Design review of the part built by this model. Coordinates are the model's own, in mm. A direction names the side the tool comes from. Coordinates: 2 decimals unless noted, no trailing zeros. Loops run counter-clockwise (first coordinate to the right, second up) from the corner with the lowest first, then second, coordinate; pieces in that order, holes last. Notation, with made-up numbers: (15, 63.5) -> (19, 63.5) arc R25 ccw to (19, 97.5) -> close; hole circle Ø5 at (38.5, 15.25). An arc over 180 degrees is marked (long way). Answer as a JSON object with one key per item and string values.
Autodesk Inventor part; units mm, degrees
ref_plane "XZ Plane" through (0, 0, 0) normal (0, 1, 0) x (-1, 0, 0)
sketch "Sketch1" plane through (0, 0, 0) normal (0, 1, 0) x (-1, 0, 0)
  line L0 (0, -8.89) -> (0, 8.89)
  line L1 (-35.56, 0) -> (35.56, 0)
  line L2 (25.4, -6.35) -> (-25.4, -6.35)
  line L3 (-25.4, -6.35) -> (-25.4, 6.35)
  line L4 (-25.4, 6.35) -> (25.4, 6.35)
  line L5 (25.4, 6.35) -> (25.4, -6.35)
  point P0 (0, 0)
  dimension "d0" = 12.7
  dimension "d1" = 6.35
  dimension "d2" = 50.8
  dimension "d3" = 25.4
extrude "Extrusion1" add sketch "Sketch1" along normal blind 4.7625
sketch "Sketch2" plane through (0, 4.7625, 0) normal (0, 1, 0) x (1, 0, 0)
  line L0 (25.4, 6.35) -> (-25.4, 6.35)
  line L1 (-25.4, 6.35) -> (-25.4, -6.35)
  line L2 (-25.4, -6.35) -> (25.4, -6.35)
  line L3 (25.4, -6.35) -> (25.4, 6.35)
  line L4 (-25.4, 2.5146) -> (-12.855, 6.35)
  line L5 (25.4, 6.35) -> (-25.4, 6.35)
  line L6 (-25.4, 6.35) -> (-25.4, -6.35)
  line L7 (-25.4, -2.5146) -> (-12.855, -6.35)
  line L8 (-12.855, 6.35) -> (-12.855, -6.35) construction
  line L9 (0, 8.89) -> (0, -8.89)
  line L10 (35.56, 0) -> (-35.56, 0)
  line L11 (-1.5875, 2.2479) -> (19.05, 2.2479)
  line L12 (19.05, 2.2479) -> (19.05, -2.2479)
  line L13 (19.05, -2.2479) -> (-1.5875, -2.2479)
  line L14 (-1.5875, -2.2479) -> (-1.5875, 2.2479)
  circle A0 centre (19.05, 0) radius 2.2479
  circle A1 centre (-1.5875, 0) radius 2.2479
  point P0 (0, 0)
  dimension "d6" = 163
  dimension "d7" = 163
  dimension "d8" = 5.0292
  dimension "d9" = 4.4958
  dimension "d10" = 6.35
  dimension "d11" = 20.6375
extrude "Extrusion2" cut sketch "Sketch2" against normal through all contours L4 L1 L0 | L11 A0 L10 A1 L9 | L9 A1 L11 | A1 L10 L9 | L9 L10 L14 A1 | L14 L10 A1 | A0 L10 L12 | L12 L10 A0 | L7 L2 L1 | L10 L14 A1 | A0 L12 L10 | L10 A1 L9 | L9 A1 L14 L10 | L10 A0 L13 L9 A1 | L12 A0 L10 | A1 L9 L13
sketch "Sketch3" plane through (0, 4.7625, 0) normal (0, 1, 0) x (1, 0, 0)
  line L0 (-25.4, -2.5146) -> (-12.855, -6.35)
  line L1 (-12.855, -6.35) -> (25.4, -6.35)
  line L2 (25.4, -6.35) -> (25.4, 6.35)
  line L3 (25.4, 6.35) -> (-12.855, 6.35)
  line L4 (-12.855, 6.35) -> (-25.4, 2.5146)
  line L5 (-25.4, 2.5146) -> (-25.4, -2.5146)
  line L6 (19.05, -2.2479) -> (-1.5875, -2.2479)
  arc A0 (-1.5875, 2.2479) -> (-1.5875, -2.2479) centre (-1.5875, 0) ccw
  line L7 (-1.5875, 2.2479) -> (19.05, 2.2479)
  arc A1 (19.05, -2.2479) -> (19.05, 2.2479) centre (19.05, 0) ccw
  line L8 (35.56, 0) -> (-35.56, 0)
  line L9 (-25.4, 1.6803) -> (-21.717, 0.762)
  line L10 (-21.717, 0.762) -> (-21.717, -0.762)
  line L11 (-21.717, -0.762) -> (-25.4, -1.6803)
  line L12 (-25.4, 2.5146) -> (-25.4, -2.5146)
  line L13 (-25.4, 1.6803) -> (-25.4, -1.6803)
  point P0 (0, 0)
  dimension "d14" = 28
  dimension "d15" = 14
  dimension "d16" = 3.683
  dimension "d17" = 1.524
  dimension "d18" = 0.762
extrude "Extrusion3" cut sketch "Sketch3" against normal blind 1.27 contours L5 L8 L10 L11 | L5 L9 L10 L8
sketch "Sketch4" plane through (0, 4.7625, 0) normal (0, 1, 0) x (1, 0, 0)
  line L0 (19.05, -2.2479) -> (-1.5875, -2.2479)
  arc A0 (-1.5875, 2.2479) -> (-1.5875, -2.2479) centre (-1.5875, 0) ccw
  line L1 (-1.5875, 2.2479) -> (19.05, 2.2479)
  arc A1 (19.05, -2.2479) -> (19.05, 2.2479) centre (19.05, 0) ccw
  line L2 (-25.4, 1.6803) -> (-21.717, 0.762)
  line L3 (-21.717, 0.762) -> (-21.717, -0.762)
  line L4 (-21.717, -0.762) -> (-25.4, -1.6803)
  line L5 (-25.4, -1.6803) -> (-25.4, -2.5146)
  line L6 (-25.4, -2.5146) -> (-12.855, -6.35)
  line L7 (-12.855, -6.35) -> (25.4, -6.35)
  line L8 (25.4, -6.35) -> (25.4, 6.35)
  line L9 (25.4, 6.35) -> (-12.855, 6.35)
  line L10 (-12.855, 6.35) -> (-25.4, 2.5146)
  line L11 (-25.4, 2.5146) -> (-25.4, 1.6803)
  line L12 (0, 8.89) -> (0, -8.89)
  line L13 (35.56, 0) -> (-35.56, 0)
  point P0 (0, 0)
  point P1 (-11.43, 0)
  dimension "d21" = 36.83
hole "Hole1" at (-11.43, 4.7625, 0) direction (0, -1, 0) diameter 3.302 depth 12.2936 tip angle 118
sketch "Sketch6" plane through (25.4, 0, 6.35) normal (0, 0, 1) x (1, 0, 0)
  line L0 (-38.255, 0) -> (-50.8, 0)
  line L1 (-38.255, 4.7625) -> (-38.255, 0)
  line L2 (-50.8, 4.7625) -> (-38.255, 4.7625)
  line L3 (-50.8, 0) -> (-50.8, 4.7625)
  line L4 (-38.255, 4.7625) -> (-38.255, 0)
  line L5 (0, 0) -> (-38.255, 0)
  line L6 (0, 0) -> (0, 4.7625)
  line L7 (-38.255, 4.7625) -> (0, 4.7625)
  line L8 (-50.8, 2.4765) -> (-42.6997, 0)
  line L9 (-50.8, 2.4765) -> (-50.8, -12.0091)
  line L10 (-50.8, -12.0091) -> (-42.6997, -12.0091)
  line L11 (-42.6997, -12.0091) -> (-42.6997, 0)
  point P0 (-25.4, 0)
  dimension "d31" = 163
  dimension "d32" = 2.286
extrude "Extrusion4" cut sketch "Sketch6" against normal through all contours L11 L10 L9 L0 | L0 L3 L8
equation "\"d1\" = 0.5 * d0"
equation "\"d3\" = 0.5 * d2"
equation "\"d7\" = d6"
equation "\"d15\" = 0.5 * d14"
equation "\"d18\" = 0.5 * d17"
properties part number "ArmBar-V03" material "Stainless Steel"
1) Add section B-B, the plane z = 0. Give the boundary of the cut face in (x, y).
Completed:
{"outline": "(-25.4, 2.48) -> (-17.3, 0) -> (-13.08, 0) -> (-13.08, 4.76) -> (-21.72, 4.76) -> (-21.72, 3.49) -> (-25.4, 3.49) -> close; (-9.78, 0) -> (-3.84, 0) -> (-3.84, 4.76) -> (-9.78, 4.76) -> close; (21.3, 0) -> (25.4, 0) -> (25.4, 4.76) -> (21.3, 4.76) -> close"}
2) Add section C-C, the plane y = 4.1. Count the separate pieces of the cut face and the enclosed holes in it, and give its area (3 significant figures).
Completed:
{"separate pieces": "1", "enclosed holes": "2", "area": "471 mm²"}
3) Wall thickness on probe 1 along X at (y, z) = (3.3, 0); probe 2 along Z at (x, y) = (14, 0.35); probe 3 along Z at (x, y) = (-11.43, 1.8): over which ranges is each line inside the solid? List them lowest first.
Completed:
{"probe 1": "-25.4 to -13.08, -9.78 to -3.84, 21.3 to 25.4", "probe 2": "-6.35 to -2.25, 2.25 to 6.35", "probe 3": "-6.35 to -1.65, 1.65 to 6.35"}
4) Add section D-D, the plane x = 0. Give the boundary of the cut face in (y, z).
Completed:
{"outline": "(0, -6.35) -> (4.76, -6.35) -> (4.76, -2.25) -> (0, -2.25) -> close; (0, 2.25) -> (4.76, 2.25) -> (4.76, 6.35) -> (0, 6.35) -> close"}
5) Clearance check with flat-ended pins moving along their axes: pin 1 Ø2.5 at (x, z) = (-11.43, 0) entering from +Y; pin 2 Ø1.5 at (x, y) = (-19, 3.5) entering from -Z; pin 3 Ø1 at (x, z) = (-24, -0.5) entering from +Y. State where each tip first meets the part, or that it passes through.
Completed:
{"pin 1": "through", "pin 2": "z = -4.7", "pin 3": "y = 3.49"}
6) For faces 1 (the flat face through (9, 2, -2.248)), 2 (the flat face through (-25.4, 3, 0)), 3 (the flat face through (-21.717, 4, 0)), list the 3-axis set-ups (+Z, -Z, +X, -X, +Y, -Y) from which the entire face can be reached by the end or side of a thin tool; tool diameter is ignored.
Completed:
{"face 1": "+Y, -Y", "face 2": "+Z, -Z, -X, +Y, -Y", "face 3": "-X, +Y"}
7) Add section A-A, the plane x = -11.43. Give the boundary of the cut face in (y, z), and give its area (3 significant figures).
Completed:
{"outline": "(0, -6.35) -> (4.76, -6.35) -> (4.76, -1.65) -> (0, -1.65) -> close; (0, 1.65) -> (4.76, 1.65) -> (4.76, 6.35) -> (0, 6.35) -> close", "area": "44.8 mm²"}
